Source: CAD feature listing. Evaluate the final solid. Frame: model axes, mm. Face numbers are marked on the shaded views. Give positions to 0.01 mm unless a question says otherwise; leave off trailing zeros. Order: outer loops, then holes, each group sorted by start corner. A loop starts at its lowest first (then second) coordinate and runs counter-clockwise, first axis right, second up.
1) Section B-B, the plane z = 11.25. Return loops of the section in (x, y) (1 decimal).
2) Section A-A, the plane z = 9.75. Return loops of the section in (x, y).
3) First-contact query: P1, Ø0.5, axis at y = 1, z = 1, coming from the +X side; P2, Ø0.5, axis at y = 0, z = 1, coming from the -X side; P3, Ø1.4, axis at x = 1.5, z = 0.5, coming from the -Y side. Flat tips, straight axial feed; report the tip coordinate or a pass-through.
4) Material intervals for line 1 (Y direction, x = -1.5, z = 1.5); line 2 (X direction, y = 1.75, z = 1.25); line 3 (X direction, y = 0, z = 9.5), sorted ascending.
5) Draft query along X for the marked faces 1, 2 and 3. Return one class per face: released by +X, released by -X, zero draft, split by the parting line, or undercut.
Autodesk Inventor part; units mm, degrees
ref_plane "CS_ANBAU_XY" through (0, 0, 0) normal (0, 0, -1) x (0, 1, 0)
ref_plane "CS_ANBAU_YZ" through (0, 0, 0) normal (0, 1, 0) x (1, 0, 0)
ref_plane "CS_ANBAU_ZX" through (0, 0, 0) normal (1, 0, 0) x (0, 0, -1)
sketch "Sketch_1" plane through (0, 0, 0) normal (1, 0, 0) x (0, 1, 0)
  line L0 (0, 0) -> (0, 12.7)
  line L1 (0, 12.7) -> (2.1, 10.7)
  line L2 (2.1, 10.7) -> (2.1, 3.263)
  line L3 (2.1, 3.263) -> (4.2, 0.6)
  line L4 (4.2, 0.6) -> (4.2, 0)
  line L5 (4.2, 0) -> (0, 0)
  line L6 (0, 0) -> (0, 12.7)
revolve "Revolution1" add sketch "Sketch_1" angle 360 about axis through (0, 0, 0) along (0, 0, -1)
sketch "Sketch_3" plane through (0, 0, 0) normal (0, 0, -1) x (0, 1, 0)
  line L0 (-2.3, -0.4905) -> (-0.4905, -0.4905)
  line L1 (-0.4905, -0.4905) -> (-0.4905, -2.3)
  line L2 (-0.4905, -2.3) -> (0.4905, -2.3)
  line L3 (0.4905, -2.3) -> (0.4905, -0.4905)
  line L4 (0.4905, -0.4905) -> (2.3, -0.4905)
  line L5 (2.3, -0.4905) -> (2.3, 0.4905)
  line L6 (2.3, 0.4905) -> (0.4905, 0.4905)
  line L7 (0.4905, 0.4905) -> (0.4905, 2.3)
  line L8 (0.4905, 2.3) -> (-0.4905, 2.3)
  line L9 (-0.4905, 2.3) -> (-0.4905, 0.4905)
  line L10 (-0.4905, 0.4905) -> (-2.3, 0.4905)
  line L11 (-2.3, 0.4905) -> (-2.3, -0.4905)
extrude "Extrusion1" cut sketch "Sketch_3" against normal blind 2
ref_plane "CS_ANBAU_XY" through (0, 0, 0) normal (0, 0, -1) x (0, 1, 0)
ref_plane "CS_ANBAU_YZ" through (0, 0, 0) normal (0, 1, 0) x (1, 0, 0)
ref_plane "CS_ANBAU_ZX" through (0, 0, 0) normal (1, 0, 0) x (0, 0, -1)
properties part number "100031"
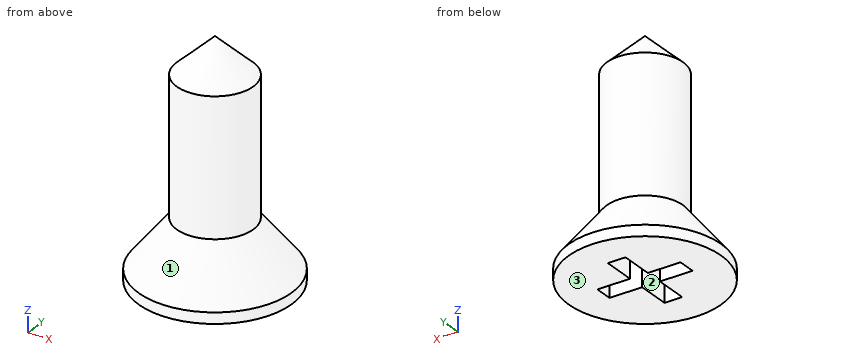
From the geometry:
1. outline: circle Ø3 at (0, 0)
2. outline: circle Ø4.2 at (0, 0)
3. P1: stops at x = 3.97
3. P2: stops at x = -4.08
3. P3: stops at y = -4.12
4. line 1: y = -3.15 to -0.49, 0.49 to 3.15
4. line 2: x = -3.25 to -0.49, 0.49 to 3.25
4. line 3: x = -2.1 to 2.1
5. face 1: split by the parting line
5. face 2: undercut
5. face 3: zero draft
